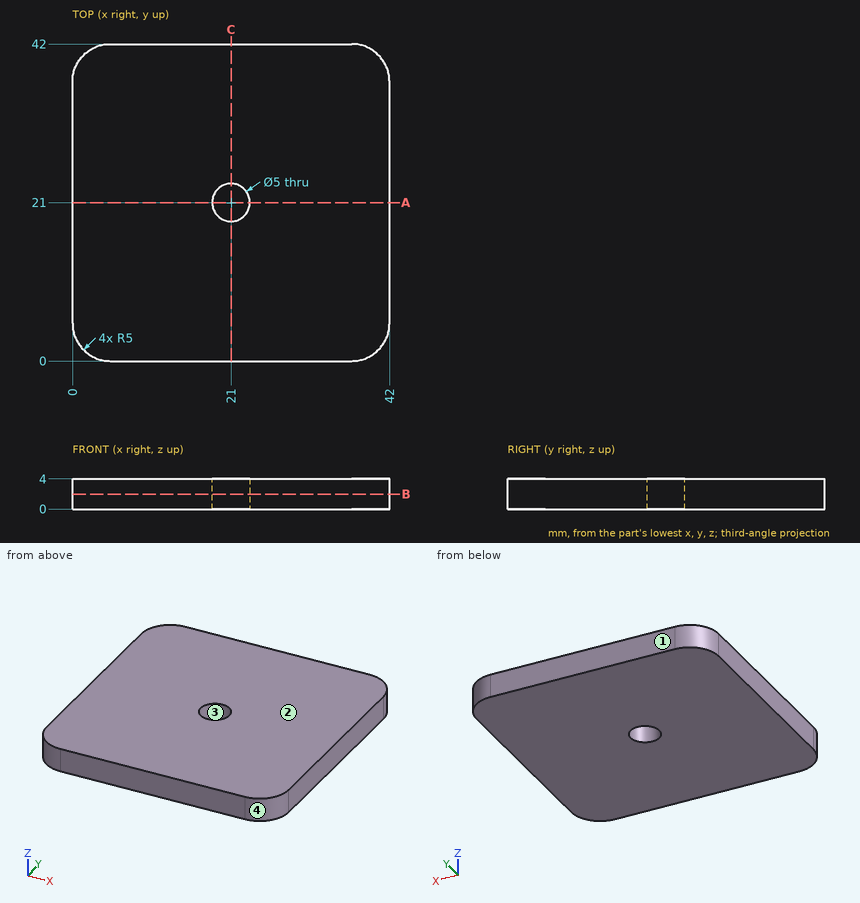
Geometry: see drawing. Coordinates: mm, zero at the bounding-box minimum. Round coordinates to 2 decimals unless told otherwise and drop trailing zeros. Order: outer loops, then holes, each group sorted by start corner. A loop starts at its lowest first (then second) coordinate and runs counter-clockwise, first axis right, second up. Notation, with made-up numbers: (30.25, 87) - (65.25, 87) arc R25 cw to (65.25, 103) - close; hole circle Ø5 at (46.5, 35.25). An arc over 180 degrees is marked (long way). One line per question, with ' | ' between items. Start each with the question number.
1) Cut plane A-A, the plane y = 21. Return the cut outline in (x, z).
2) Cut plane B-B, the plane z = 2. Return the cut outline in (x, y), then the cut area to 3 significant figures.
3) Ray query, probe 1 along Y at (x, z) = (21, 2.3); probe 2 along X at (y, z) = (40, 0.3); probe 3 along Y at (x, z) = (4, 0.5). Return the intervals inside material, ascending.
4) Pull-direction query (Y, two-part tool) for the marked faces 1, 2, 3 and 4; classes: +Y half, -Y half, draft (parallel to the pull), parting line (faces both ways), or undercut.
Worked out:
1) outline: (0, 0) - (18.5, 0) - (18.5, 4) - (0, 4) - close; (23.5, 0) - (42, 0) - (42, 4) - (23.5, 4) - close
2) outline: (0, 5) arc R5 ccw to (5, 0) - (37, 0) arc R5 ccw to (42, 5) - (42, 37) arc R5 ccw to (37, 42) - (5, 42) arc R5 ccw to (0, 37) - close; hole circle Ø5 at (21, 21) | area: 1,720 mm^2
3) probe 1: y = 0 to 18.5, 23.5 to 42 | probe 2: x = 1 to 41 | probe 3: y = 0.1 to 41.9
4) face 1: +Y half | face 2: draft | face 3: undercut | face 4: -Y half
